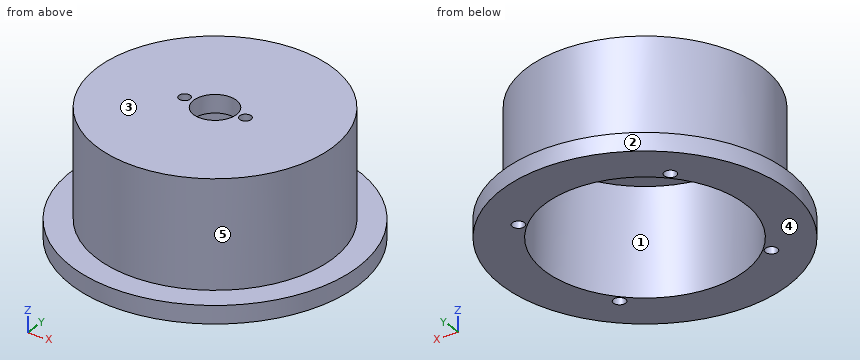
from build123d import *

# Parameters (mm, degrees)
SKETCH1_R           = 40
SKETCH1_R_2         = 28
FLANGE_DEPTH        = 5
SKETCH2_R           = 33
SKETCH2_R_2         = 28
TUBE_DEPTH          = 25
SKETCH3_R           = 33
PLATE_DEPTH         = 5
SKETCH4_R           = 6
SHAFT_HOLE_DEPTH    = 5
SKETCH5_R           = 1.6
MOTOR_SCREWS_DEPTH  = 5
SKETCH6_R           = 1.7
GROMMET_HOLES_DEPTH = 5


with BuildPart() as part:
    # Sketch1 → Flange (new body)
    with BuildSketch(Plane.XY):
        Circle(SKETCH1_R)
        Circle(SKETCH1_R_2, mode=Mode.SUBTRACT)
    extrude(amount=FLANGE_DEPTH)

    # Sketch2 → Tube (add)
    with BuildSketch(Plane.XY.offset(5)):
        Circle(SKETCH2_R)
        Circle(SKETCH2_R_2, mode=Mode.SUBTRACT)
    extrude(amount=TUBE_DEPTH)

    # Sketch3 → Plate (add)
    with BuildSketch(Plane.XY.offset(30)):
        Circle(SKETCH3_R)
    extrude(amount=PLATE_DEPTH)

    # Sketch4 → Shaft_hole (cut)
    with BuildSketch(Plane.XY.offset(30)):
        Circle(SKETCH4_R)
    extrude(amount=SHAFT_HOLE_DEPTH, mode=Mode.SUBTRACT)

    # Sketch5 → Motor_screws (cut)
    with BuildSketch(Plane.XY.offset(30)):
        with Locations((-8.5, 0)):
            Circle(SKETCH5_R)
        with Locations((8.5, 0)):
            Circle(SKETCH5_R)
    extrude(amount=MOTOR_SCREWS_DEPTH, mode=Mode.SUBTRACT)

    # Sketch6 → Grommet_holes (cut)
    with BuildSketch(Plane.XY):
        with Locations((21.213203436, 21.213203436)):
            Circle(SKETCH6_R)
        with Locations((-21.213203436, 21.213203436)):
            Circle(SKETCH6_R)
        with Locations((-21.213203436, -21.213203436)):
            Circle(SKETCH6_R)
        with Locations((21.213203436, -21.213203436)):
            Circle(SKETCH6_R)
    extrude(amount=GROMMET_HOLES_DEPTH, mode=Mode.SUBTRACT)


solid = part.part
CAD build for the part. Positions are in the model's coordinates, mm. Face numbers are marked on the shaded views. A direction names the side the tool comes from. Round coordinates to 2 decimals unless told otherwise and drop trailing zeros. Write each loop counter-clockwise with the first axis right and the second up, starting at its lowest first coordinate (ties: lowest second). Pieces come first, ordered by that corner, then holes.
(1) Slice it at C-C, the plane y = -18.5. Write the cut outline in (x, z).
(2) Slice it at B-B, the plane x = 0. Write the cut outline in (y, z).
(3) Probe line 1 along Y through (x, z) = (0, 16.5); line 2 along Z through (x, y) = (31.5, 10.5). List the from-to ranges inside material, lowest first.
(4) Slice it at D-D, the plane x = 8.5. Write the cut outline in (y, z), and give its area (3 significant figures).
(5) Drop flat-ended pins along their axis: P1, Ø2, axis at x = 17, z = 10, coming from the -Y side; P2, Ø12, axis at x = 14, z = 24, coming from the -Y side; P3, Ø2.5, axis at x = -21, y = -21.5, coming from the -Z side. Give the stop position or say it passes through.
(6) Mould opens along Y. For the marked faces 1, 2 and 3 say: pulls with the +Y half, pulls with the -Y half, needs draft (parallel to the pull), parting line crosses it, or undercut.
(7) Slice it at A-A, the plane y = 0. Write the cut outline in (x, z), and give its area (3 significant figures).
(8) 3-axis set-ups, long thin cutter, end or side, ignore diameter. For the marked faces 4 and 5: which of +Z, -Z, +X, -X, +Y, -Y reach the whole face in a straight line?
From the geometry:
1. outline: (-35.46, 0) - (-21.02, 0) - (-21.02, 30) - (21.02, 30) - (21.02, 0) - (35.46, 0) - (35.46, 5) - (27.33, 5) - (27.33, 35) - (-27.33, 35) - (-27.33, 5) - (-35.46, 5) - close
2. outline: (-40, 0) - (-28, 0) - (-28, 30) - (-6, 30) - (-6, 35) - (-33, 35) - (-33, 5) - (-40, 5) - close; (6, 30) - (28, 30) - (28, 0) - (40, 0) - (40, 5) - (33, 5) - (33, 35) - (6, 35) - close
3. line 1: y = -33 to -28, 28 to 33
3. line 2: z = 0 to 5
4. outline: (-39.09, 0) - (-26.68, 0) - (-26.68, 30) - (-1.6, 30) - (-1.6, 35) - (-31.89, 35) - (-31.89, 5) - (-39.09, 5) - close; (1.6, 30) - (26.68, 30) - (26.68, 0) - (39.09, 0) - (39.09, 5) - (31.89, 5) - (31.89, 35) - (1.6, 35) - close
4. area: 687 mm2
5. P1: stops at y = -28.86
5. P2: stops at y = -32.02
5. P3: stops at z = 5
6. face 1: undercut
6. face 2: parting line crosses it
6. face 3: needs draft
7. outline: (-40, 0) - (-28, 0) - (-28, 30) - (-10.1, 30) - (-10.1, 35) - (-33, 35) - (-33, 5) - (-40, 5) - close; (-6.9, 30) - (-6, 30) - (-6, 35) - (-6.9, 35) - close; (6, 30) - (6.9, 30) - (6.9, 35) - (6, 35) - close; (10.1, 30) - (28, 30) - (28, 0) - (40, 0) - (40, 5) - (33, 5) - (33, 35) - (10.1, 35) - close
7. area: 608 mm2
8. face 4: -Z, +X, -X, +Y, -Y
8. face 5: +Z
